from build123d import *

# Parameters (mm, degrees)
SKETCH1_R               = 7.5
BOSS_EXTRUDE1_DEPTH     = 10
BOSS_EXTRUDE2_DEPTH     = 3.4
BOSS_EXTRUDE3_DEPTH     = 7
CUT_EXTRUDE1_DEPTH      = 38.901187316
CUT_EXTRUDE1_DEPTH_BACK = 38.901187316
SKETCH4_R               = 1.5
SKETCH5_R               = 4
CUT_EXTRUDE2_DEPTH      = 31.041637772
CUT_EXTRUDE3_DEPTH      = 37.675059645
CUT_EXTRUDE3_DEPTH_BACK = 37.675059645
SKETCH6_R               = 1.25


with BuildPart() as part:
    # Sketch1 → Boss-Extrude1 (new body)
    with BuildSketch(Plane(origin=(0, 0, 0), x_dir=(0, 0, -1), z_dir=(1, 0, 0))):
        Circle(SKETCH1_R)
    extrude(amount=BOSS_EXTRUDE1_DEPTH)

    # Sketch2 → Boss-Extrude2 (add, symmetric)
    with BuildSketch(Plane.XY):
        with BuildLine():
            Line((0, 0), (0, 9.115122314))
            ThreePointArc((0, 9.115122314), (0.188996508, 9.963807387), (0.720266353, 10.652093944))
            Line((0.720266353, 10.652093944), (17.440532706, 24.573943261))
            ThreePointArc((17.440532706, 24.573943261), (23.073943261, 24.059467294), (22.559467294, 18.426056739))
            Line((22.559467294, 18.426056739), (10.360133176, 8.268485815))
            ThreePointArc((10.360133176, 8.268485815), (10.094498254, 7.924342536), (10, 7.5))
            Line((10, 7.5), (10, 0))
            Line((10, 0), (0, 0))
        make_face()
    extrude(amount=BOSS_EXTRUDE2_DEPTH, both=True)

    # Sketch3 → Boss-Extrude3 (add, symmetric)
    with BuildSketch(Plane.XY):
        with BuildLine():
            Line((9, -9.5), (9, 0))
            Line((9, 0), (0, 0))
            Line((0, 0), (0, -9.5))
            ThreePointArc((0, -9.5), (4.5, -14), (9, -9.5))
        make_face()
    extrude(amount=BOSS_EXTRUDE3_DEPTH, both=True)

    # Sketch4 → Cut-Extrude1 (cut, two sides: drawn at the far end of the back side and taken through both)
    with BuildSketch(Plane.XY.offset(7).offset(-CUT_EXTRUDE1_DEPTH_BACK)):
        with Locations((4.5, -9.5)):
            Circle(SKETCH4_R)
    extrude(amount=CUT_EXTRUDE1_DEPTH + CUT_EXTRUDE1_DEPTH_BACK, mode=Mode.SUBTRACT)

    # Sketch5 → Cut-Extrude2 (cut, through all)
    with BuildSketch(Plane(origin=(10, 0, 0), x_dir=(0, 0, -1), z_dir=(1, 0, 0))):
        Circle(SKETCH5_R)
    extrude(amount=-CUT_EXTRUDE2_DEPTH, mode=Mode.SUBTRACT)

    # Sketch6 → Cut-Extrude3 (cut, two sides: drawn at the far end of the back side and taken through both)
    with BuildSketch(Plane.XY.offset(3.4).offset(-CUT_EXTRUDE3_DEPTH_BACK)):
        with Locations((20, 21.5)):
            Circle(SKETCH6_R)
    extrude(amount=CUT_EXTRUDE3_DEPTH + CUT_EXTRUDE3_DEPTH_BACK, mode=Mode.SUBTRACT)


solid = part.part
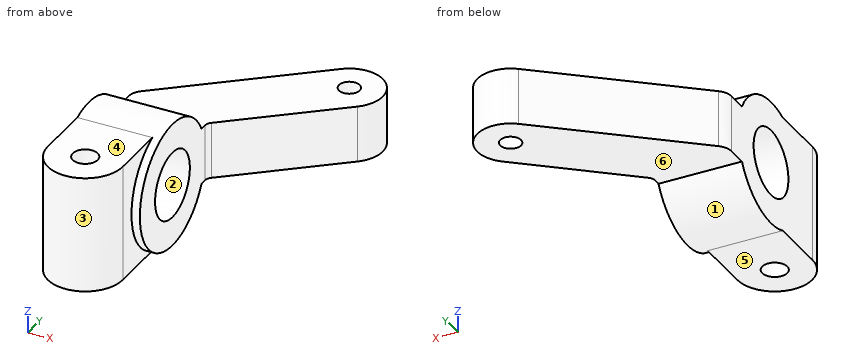
Source: CAD feature listing. Evaluate the final solid. Frame: model axes, mm. Face numbers are marked on the shaded views. A direction names the side the tool comes from. Round coordinates to 2 decimals unless told otherwise and drop trailing zeros. Order: outer loops, then holes, each group sorted by start corner. A loop starts at its lowest first (then second) coordinate and runs counter-clockwise, first axis right, second up. Notation, with made-up numbers: (-6, -33) - (8, -33) arc R24 cw to (8, -14) - close; hole circle Ø8 at (-27.75, 23). An arc over 180 degrees is marked (long way). Use a Markdown table: item, result. Add a question column.
1. Line query: probe 1 along Y at (x, z) = (3.75, 1); probe 2 along Y at (x, z) = (20, -0.5); probe 3 along Y at (x, z) = (7.75, 0). Output: solid intervals per line, ascending.
2. First-contact query: pin 1 (3 mm diameter, centred on x = 20, y = 21.5, fed in from -Z); pin 2 (4 mm diameter, centred on y = 18.5, z = -5, fed in from -X); pin 3 (2 mm diameter, centred on x = 9.5, z = 2.5, fed in from -Y); pin 4 (6 mm diameter, centred on y = 20.5, z = 5, fed in from +X). Flat tips, straight axial feed; report the tip coordinate or a pass-through.
3. Section query A-A (z = 0.25). Return the cut outline in (x, y).
4. Section query B-B (x = 4). Return the cut outline in (y, z), then the cut area to 3 significant figures.
5. Section query C-C (y = 21.5). Return the cut outline in (x, z), then the cut area to 3 significant figures.
6. Section query D-D (z = 6). Return the cut outline in (x, y).
7. Set-up query: the marked faces 4, 5 and 6. Return all of +Z, -Z, +X, -X, +Y, -Y with unobstructed straight access to the full face (end or side cutting, diameter ignored); none if empty.
8. Mould query, pull axis Y, two halves, no side actions, for the marked faces 1, 2 and 3. Classes: +Y half, -Y half, draft (parallel to the pull), parting line (faces both ways), or undercut.
Derived:
| question | item | result |
|---|---|---|
| 1 | probe 1 | -13.94 to -10.8, -8.2 to -3.87, 3.87 to 13.17 |
| 1 | probe 2 | 16.29 to 20.25, 22.75 to 25.5 |
| 1 | probe 3 | -12.61 to -4, 4 to 16.51 |
| 2 | pin 1 | z = -3.4 |
| 2 | pin 2 | x = 8.7 |
| 2 | pin 3 | y = -11.56 |
| 2 | pin 4 | x = 24 |
| 3 | outline | (0, -9.5) arc R4.5 ccw to (9, -9.5) - (9, -7.5) - (10, -7.5) - (10, -3.99) - (0, -3.99) - close; (0, 3.99) - (10, 3.99) - (10, 7.5) arc R1 cw to (10.36, 8.27) - (22.56, 18.43) arc R4 ccw to (17.44, 24.57) - (0.72, 10.65) arc R2 ccw to (0, 9.12) - close; hole circle Ø3 at (4.5, -9.5); hole circle Ø2.5 at (20, 21.5) |
| 4 | outline | (-13.97, -7) - (-10.91, -7) - (-10.91, 7) - (-13.97, 7) - close; (-8.09, -7) - (-2.69, -7) arc R7.5 ccw to (6.69, -3.4) - (13.38, -3.4) - (13.38, 3.4) - (6.69, 3.4) arc R7.5 ccw to (-2.69, 7) - (-8.09, 7) - close; hole circle Ø8 at (0, 0) |
| 4 | area | 238 mm2 |
| 5 | outline | (13.75, -3.4) - (18.75, -3.4) - (18.75, 3.4) - (13.75, 3.4) - close; (21.25, -3.4) - (24, -3.4) - (24, 3.4) - (21.25, 3.4) - close |
| 5 | area | 52.7 mm2 |
| 6 | outline | (0, -9.5) arc R4.5 ccw to (9, -9.5) - (9, -4.5) - (10, -4.5) - (10, 4.5) - (0, 4.5) - close; hole circle Ø3 at (4.5, -9.5) |
| 7 | face 4 | +Z, +X, -X, -Y |
| 7 | face 5 | -Z, +X, -X, -Y |
| 7 | face 6 | -Z, +X, -X, +Y |
| 8 | face 1 | parting line |
| 8 | face 2 | undercut |
| 8 | face 3 | -Y half |
